Design review of the part built by this model. Coordinates are the model's own, in mm. Face numbers are marked on the shaded views. A direction names the side the tool comes from. Round coordinates to 2 decimals unless told otherwise and drop trailing zeros. Loops run counter-clockwise (first coordinate to the right, second up) from the corner with the lowest first, then second, coordinate; pieces in that order, holes last. Notation, with made-up numbers: (44, 13.25) - (69, 13.25) arc R19 cw to (69, 35.25) - close; hole circle Ø1 at (23.5, 68). An arc over 180 degrees is marked (long way). Return JSON: item names as keys, results as strings. Group by question number.
(1) Wall thickness on L1, parallel to X at y = 14.5, z = 42; L2, parallel to Z at x = -91, y = 12.5; L3, parallel to Z at x = -59.5, y = 2: over which ranges is each line inside the solid? List them lowest first. Write a range as [from, to].
(2) Clearance check with flat-ended pins moving along their axes: pin 1 (12 mm diameter, centred on y = -1, z = 47.5, fed in from -X); pin 2 (17.5 mm diameter, centred on x = -84.5, y = 4.5, fed in from -Z). State where each tip first meets the part, or that it passes through.
(3) We need section D-D, the plane y = -9.5. Write out the cut boundary in (x, z), and give its area (3 significant figures).
(4) We need section A-A, the plane y = 2.5. Write out the cut boundary in (x, z).
(5) We need section C-C, the plane z = 56. Write out the cut boundary in (x, y).
(6) For the marked faces 1 and 2, list the 3-axis set-ups (+Z, -Z, +X, -X, +Y, -Y) from which the entire face can be reached by the end or side of a thin tool; tool diameter is ignored.
(7) We need section B-B, the plane x = -69.5. Write out the cut boundary in (y, z), and give its area (3 significant figures).
from build123d import *

# Parameters (mm, degrees)
BOSS_EXTRUDE1_DEPTH = 20
SKETCH2_R           = 5
CUT_EXTRUDE1_DEPTH  = 40
FILLET1_R           = 20
FILLET2_R           = 20


with BuildPart() as part:
    # Sketch1 → Boss-Extrude1 (new, symmetric)
    with BuildSketch(Plane(origin=(0, 0, 0), x_dir=(1, 0, 0), z_dir=(0, 1, 0))):
        Polygon((-56.045207575, 13.418938385), (-61.045207575, 13.418938385), (-61.045207575, -76.581061615), (-96.045207575, -76.581061615), (-96.045207575, -81.581061615), (-56.045207575, -81.581061615), align=None)
    extrude(amount=BOSS_EXTRUDE1_DEPTH, both=True)

    # Sketch2 → Cut-Extrude1 (cut)
    with BuildSketch(Plane.ZY.offset(61.045207575)):
        with Locations((6.581061615, 0)):
            Circle(SKETCH2_R)
    extrude(amount=-CUT_EXTRUDE1_DEPTH, mode=Mode.SUBTRACT)

    # Fillet1
    fillet1_edges = [part.edges().sort_by_distance(p)[0] for p in [
        (-58.545207575, 20, -13.418938385),
    ]]
    fillet(fillet1_edges, radius=FILLET1_R)

    # Fillet2
    fillet2_edges = [part.edges().sort_by_distance(p)[0] for p in [
        (-58.545207575, -20, -13.418938385),
    ]]
    fillet(fillet2_edges, radius=FILLET2_R - 0.0001)  # a hair under: the kernel refuses the full size


solid = part.part
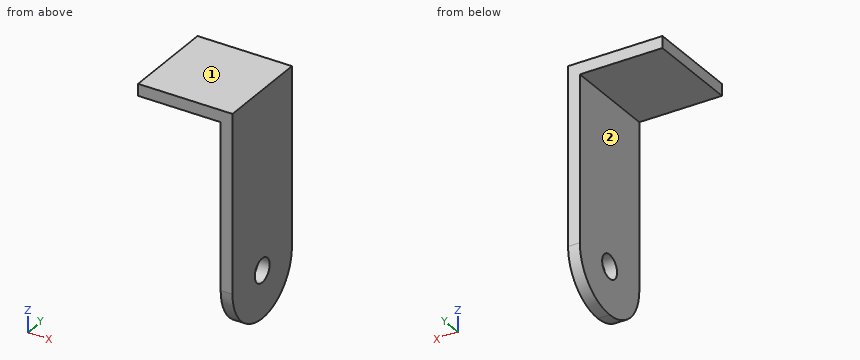
Solutions:
{
 "1": {"L1": "[-61.05, -56.05]", "L2": "[76.58, 81.58]", "L3": "[-13.32, 2], [11.16, 81.58]"},
 "2": {"pin 1": "x = -61.05", "pin 2": "z = 76.58"},
 "3": {"outline": "(-96.05, 76.58) - (-61.05, 76.58) - (-61.05, -11.02) - (-56.05, -11.02) - (-56.05, 81.58) - (-96.05, 81.58) - close", "area": "638 mm^2"},
 "4": {"outline": "(-96.05, 76.58) - (-61.05, 76.58) - (-61.05, 10.91) - (-56.05, 10.91) - (-56.05, 81.58) - (-96.05, 81.58) - close; (-61.05, -13.26) - (-56.05, -13.26) - (-56.05, 2.25) - (-61.05, 2.25) - close"},
 "5": {"outline": "(-61.05, -20) - (-56.05, -20) - (-56.05, 20) - (-61.05, 20) - close"},
 "6": {"face 1": "+Z, +X, -X, +Y, -Y", "face 2": "-Z, -X, +Y, -Y"},
 "7": {"outline": "(-20, 76.58) - (20, 76.58) - (20, 81.58) - (-20, 81.58) - close", "area": "200 mm^2"}
}
